Part print with two shaded views. Sizes in mm from the minimum x, y, z corner. Coordinates: 2 decimals unless noted, no trailing zeros. Loops run counter-clockwise (first coordinate to the right, second up) from the corner with the lowest first, then second, coordinate; pieces in that order, holes last. Notation, with made-up numbers: (49.25, 10) -> (108.25, 10) arc R27 ccw to (108.25, 49) -> close; hole circle Ø4 at (56, 70). An arc over 180 degrees is marked (long way). Write each question's results on one line, items separated by ' | '.
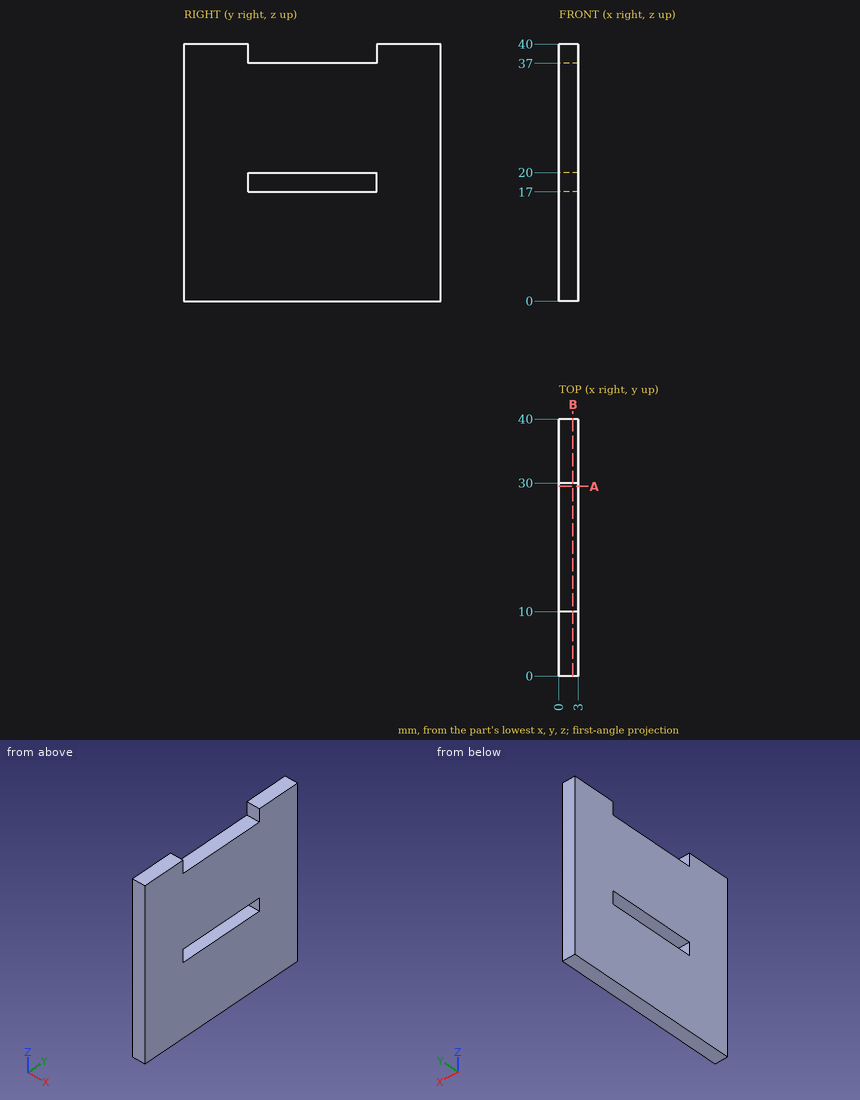
Q1. Cut at A-A on y = 29.5. Write the cut outline in (x, z), and give its area (3 significant figures).
Results are:
outline: (0, 0) -> (3, 0) -> (3, 17) -> (0, 17) -> close; (0, 20) -> (3, 20) -> (3, 37) -> (0, 37) -> close | area: 102 mm^2
Q2. Drop a flat-ended pin along its axis: pin 1 (1.5 mm diameter, centred on x = 2, y = 18, fed in from +Z). Give the stop position or say it passes through.
Results are:
pin 1: z = 37
Q3. Cut at B-B on x = 2.2. Write the cut outline in (y, z).
Results are:
outline: (0, 0) -> (40, 0) -> (40, 40) -> (30, 40) -> (30, 37) -> (10, 37) -> (10, 40) -> (0, 40) -> close; hole (10, 17) -> (30, 17) -> (30, 20) -> (10, 20) -> close
Q4. Wall check: L1, parallel to Y at x = 1.7, z = 38; L2, parallel to Z at x = 1.45, y = 15. Give the ranges that are in metal, low to high. Write a range as from..to.
Results are:
L1: 0..10, 30..40 | L2: 0..17, 20..37
